Autodesk Inventor part; units mm, degrees
ref_plane "YZ Plane" through (0, 0, 0) normal (1, 0, 0) x (0, 1, 0)
ref_plane "XZ Plane" through (0, 0, 0) normal (0, 1, 0) x (-1, 0, 0)
ref_plane "XY Plane" through (0, 0, 0) normal (0, 0, 1) x (1, 0, 0)
sketch "Эскиз1" plane through (0, 0, 0) normal (0, 1, 0) x (-1, 0, 0)
  line L0 (18.1, 35) -> (-18.1, 35)
  line L1 (-18.1, 35) -> (-18.1, -35)
  line L2 (-18.1, -35) -> (18.1, -35)
  line L3 (18.1, -35) -> (18.1, 35)
  line L4 (18.1, 35) -> (-18.1, -35) construction
  line L5 (15.1, 31) -> (15.1, -31)
  line L6 (0, 0) -> (5, 0) construction
  circle A0 centre (15.1, 31) radius 1.5
  line L7 (0, 0) -> (0, 5) construction
  line L8 (0, 0) -> (3, -3) construction
  circle A1 centre (-15.1, 31) radius 1.5
  circle A2 centre (15.1, -31) radius 1.5
  circle A3 centre (-15.1, -31) radius 1.5
  point P0 (15.1, 0)
  point P1 (-15.5, 0)
  dimension "d0" = 36.2
  dimension "d1" = 70
  dimension "d2" = 4
  dimension "d3" = 3
  dimension "d4" = 3
extrude "Выдавливание1" add sketch "Эскиз1" along normal blind 16
properties part number "boost"
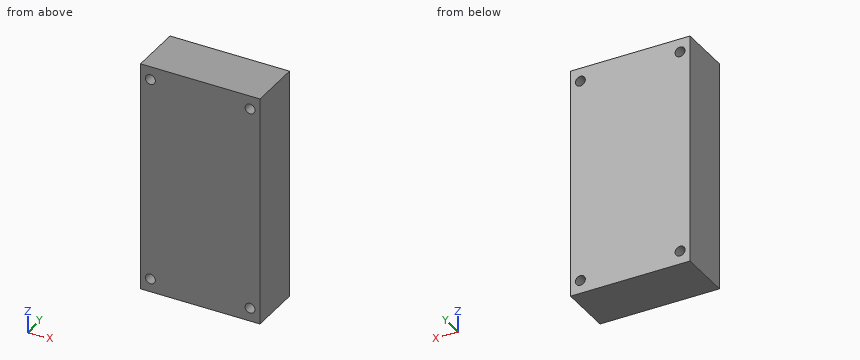
Geometry: final body of the model. Coordinates: model frame, mm. Give positions to 0.01 mm unless a question says otherwise; leave off trailing zeros. Loops run counter-clockwise (first coordinate to the right, second up) from the corner with the lowest first, then second, coordinate; pieces in that order, holes last. Notation, with made-up numbers: (-36, -28.5) -> (-1, -28.5) arc R20 ccw to (-1, -18.5) -> close; hole circle Ø10 at (-38.75, 1.25). An arc over 180 degrees is marked (long way). Return JSON: item names as keys, results as strings.
Item 1: Pin query (flat end, axial travel): P1, Ø2.5, axis at x = 15.1, z = -31, coming from the -Y side; P2, Ø4, axis at x = -15.1, z = -31, coming from the -Y side. Return the tip coordinate at first contact, or that it passes through.
Filled in:
{"P1": "through", "P2": "y = 0"}
Item 2: Section A-A, the plane x = 15.1. Output: boundary loops of the cut face in (y, z), plus the area to 3 significant figures.
Filled in:
{"outline": "(0, -35) -> (16, -35) -> (16, -32.5) -> (0, -32.5) -> close; (0, -29.5) -> (16, -29.5) -> (16, 29.5) -> (0, 29.5) -> close; (0, 32.5) -> (16, 32.5) -> (16, 35) -> (0, 35) -> close", "area": "1,020 mm^2"}
Item 3: Line query: line 1 (Z direction, x = -15.1, y = 11.5); line 2 (Z direction, x = 14, y = 7). Output: solid intervals per line, ascending.
Filled in:
{"line 1": "-35 to -32.5, -29.5 to 29.5, 32.5 to 35", "line 2": "-35 to -32.02, -29.98 to 29.98, 32.02 to 35"}
Item 4: Section B-B, the plane z = 31. Output: boundary loops of the cut face in (x, y), plus the area to 3 significant figures.
Filled in:
{"outline": "(-18.1, 0) -> (-16.6, 0) -> (-16.6, 16) -> (-18.1, 16) -> close; (-13.6, 0) -> (13.6, 0) -> (13.6, 16) -> (-13.6, 16) -> close; (16.6, 0) -> (18.1, 0) -> (18.1, 16) -> (16.6, 16) -> close", "area": "483 mm^2"}
